The model under review builds one solid part; all positions refer to its coordinate system, in mm. Face numbers are marked on the shaded views. A direction names the side the tool comes from. Coordinates: 2 decimals unless noted, no trailing zeros. Loops run counter-clockwise (first coordinate to the right, second up) from the corner with the lowest first, then second, coordinate; pieces in that order, holes last. Notation, with made-up numbers: M 81,20.25 L 117,20.25 A33 cw 117,58.25 Z; hole C 44.5,76.25 d8. An arc over 180 degrees is marked long. Use one line per item in the form item = value.
```python
from build123d import *

# Parameters (mm, degrees)
SKETCH5_R          = 4.5
CUT_EXTRUDE1_DEPTH = 86
SKETCH6_R          = 13
CUT_EXTRUDE2_DEPTH = 8
CUT_EXTRUDE4_DEPTH = 3
SKETCH9_R          = 1
CUT_EXTRUDE5_DEPTH = 5


with BuildPart() as part:
    # Sketch3 → Revolve1 (revolve)
    with BuildSketch(Plane(origin=(0, 0, 0), x_dir=(0, 0, -1), z_dir=(1, 0, 0))):
        Polygon((-24.411764706, 0), (-24.411764706, -109.5), (-19.411764706, -109.5), (-19.411764706, -94.5), (55.588235294, -94.5), (55.588235294, -109.5), (60.588235294, -109.5), (60.588235294, -84.5), (-14.411764706, -84.5), (-14.411764706, 0), align=None)
    revolve(axis=Axis((0, 0, 33.897058824), (0, 0, -1)))

    # Sketch5 → Cut-Extrude1 (cut, through all)
    with BuildSketch(Plane.XY.offset(24.411764706)):
        Circle(SKETCH5_R)
    extrude(amount=-CUT_EXTRUDE1_DEPTH, mode=Mode.SUBTRACT)

    # Sketch6 → Cut-Extrude2 (cut)
    with BuildSketch(Plane(origin=(0, 0, 14.411764706), x_dir=(-1, 0, 0), z_dir=(0, 0, -1))):
        Circle(SKETCH6_R)
    extrude(amount=-CUT_EXTRUDE2_DEPTH, mode=Mode.SUBTRACT)

    # Sketch8 → Cut-Extrude4 (cut)
    with BuildSketch(Plane(origin=(0, 0, -60.588235294), x_dir=(-1, 0, 0), z_dir=(0, 0, -1))):
        with BuildLine():
            ThreePointArc((11.969710732, 83.647928994), (0, 96.5), (-11.969710732, 83.647928994))
            ThreePointArc((-11.969710732, 83.647928994), (0, 84.5), (11.969710732, 83.647928994))
        make_face()
        with BuildLine():
            ThreePointArc((78.426086849, 31.457890927), (83.571451465, 48.25), (66.456376117, 52.190038067))
            ThreePointArc((66.456376117, 52.190038067), (73.17914662, 42.25), (78.426086849, 31.457890927))
        make_face()
        with BuildLine():
            ThreePointArc((66.456376117, -52.190038067), (83.571451465, -48.25), (78.426086849, -31.457890927))
            ThreePointArc((78.426086849, -31.457890927), (73.17914662, -42.25), (66.456376117, -52.190038067))
        make_face()
        with BuildLine():
            ThreePointArc((-11.969710732, -83.647928994), (0, -96.5), (11.969710732, -83.647928994))
            ThreePointArc((11.969710732, -83.647928994), (0, -84.5), (-11.969710732, -83.647928994))
        make_face()
        with BuildLine():
            ThreePointArc((-78.426086849, -31.457890927), (-83.571451465, -48.25), (-66.456376117, -52.190038067))
            ThreePointArc((-66.456376117, -52.190038067), (-73.17914662, -42.25), (-78.426086849, -31.457890927))
        make_face()
        with BuildLine():
            ThreePointArc((-66.456376117, 52.190038067), (-83.571451465, 48.25), (-78.426086849, 31.457890927))
            ThreePointArc((-78.426086849, 31.457890927), (-73.17914662, 42.25), (-66.456376117, 52.190038067))
        make_face()
    extrude(amount=-CUT_EXTRUDE4_DEPTH, mode=Mode.SUBTRACT)

    # Sketch9 → Cut-Extrude5 (cut)
    with BuildSketch(Plane(origin=(0, 0, -57.588235294), x_dir=(-1, 0, 0), z_dir=(0, 0, -1))):
        with Locations((0, 90.5)):
            Circle(SKETCH9_R)
        with Locations((78.375299042, 45.25)):
            Circle(SKETCH9_R)
        with Locations((78.375299042, -45.25)):
            Circle(SKETCH9_R)
        with Locations((0, -90.5)):
            Circle(SKETCH9_R)
        with Locations((-78.375299042, -45.25)):
            Circle(SKETCH9_R)
        with Locations((-78.375299042, 45.25)):
            Circle(SKETCH9_R)
    extrude(amount=-CUT_EXTRUDE5_DEPTH, mode=Mode.SUBTRACT)


solid = part.part
```
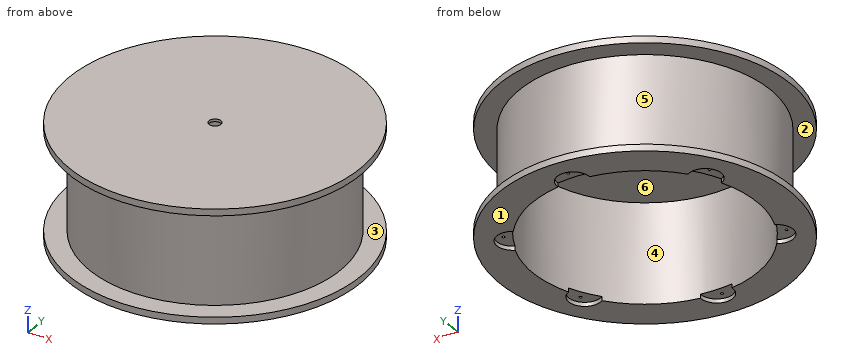
1. Add section C-C (z = -18.5). State the section outline as (x, y) points, then the cut area to 3 significant figures.
Response values:
outline = C 0,0 d189; hole C 0,0 d169
area = 5,620 mm^2
2. Add section D-D (y = 63). State the section outline as (x, z) points.
Response values:
outline = M -89.56,-60.59 L -56.31,-60.59 L -56.31,14.41 L 56.31,14.41 L 56.31,-60.59 L 89.56,-60.59 L 89.56,-55.59 L 70.44,-55.59 L 70.44,19.41 L 89.56,19.41 L 89.56,24.41 L -89.56,24.41 L -89.56,19.41 L -70.44,19.41 L -70.44,-55.59 L -89.56,-55.59 Z
3. Add section B-B (x = -8). State the section outline as (y, z) points.
Response values:
outline = M -109.21,-60.59 L -93.44,-60.59 L -93.44,-57.59 L -84.12,-57.59 L -84.12,14.41 L -10.25,14.41 L -10.25,22.41 L 10.25,22.41 L 10.25,14.41 L 84.12,14.41 L 84.12,-57.59 L 93.44,-57.59 L 93.44,-60.59 L 109.21,-60.59 L 109.21,-55.59 L 94.16,-55.59 L 94.16,19.41 L 109.21,19.41 L 109.21,24.41 L -109.21,24.41 L -109.21,19.41 L -94.16,19.41 L -94.16,-55.59 L -109.21,-55.59 Z
4. Wall thickness on line 1 along Z through (x, y) = (59.5, 88); line 2 along X through (y, z) = (-45, -54); line 3 along Y through (x, z) = (-38, -52): over which ranges is each line inside the solid? List them lowest first. Write a range as from..to.
Response values:
line_1 = -60.59..-55.59, 19.41..24.41
line_2 = -83.1..-79.34, -77.41..-71.52, 71.52..77.41, 79.34..83.1
line_3 = -86.52..-75.47, 75.47..86.52
5. Machinability: for the marked faces 1 and 2, which of the approach directions +Z, -Z, +X, -X, +Y, -Y give a long, thin tool a straight path to every point of the face, cutting with its end or side? Answer none if there is none.
Response values:
face_1 = -Z, +X, -X, +Y, -Y
face_2 = none
6. Add section A-A (y = 0). State the section outline as (x, z) points, then the cut area to 3 significant figures.
Response values:
outline = M -109.5,-60.59 L -84.5,-60.59 L -84.5,14.41 L -13,14.41 L -13,22.41 L -4.5,22.41 L -4.5,24.41 L -109.5,24.41 L -109.5,19.41 L -94.5,19.41 L -94.5,-55.59 L -109.5,-55.59 Z; M 4.5,22.41 L 13,22.41 L 13,14.41 L 84.5,14.41 L 84.5,-60.59 L 109.5,-60.59 L 109.5,-55.59 L 94.5,-55.59 L 94.5,19.41 L 109.5,19.41 L 109.5,24.41 L 4.5,24.41 Z
area = 3,460 mm^2
7. The part is to be moulded in two halves that separate along X. For the marked faces 3, 4, 5 and 6, say which applies: pulls with the +X half, pulls with the -X half, needs draft (parallel to the pull), parting line crosses it, or undercut.
Response values:
face_3 = needs draft
face_4 = undercut
face_5 = parting line crosses it
face_6 = undercut
8. Insertion check: P1, Ø0.6, axis at x = 0, y = 90, coming from the -Z side; P2, Ø2, axis at x = 27, z = -23.5, coming from the +Y side; P3, Ø6, axis at y = -78.5, z = 11.5, coming from the +X side; P4, Ø10.5, axis at x = 4, y = -91, coming from the -Z side. Each pin has a flat end and moves straight along its axis. Give the tip position at first contact, or say it passes through.
Response values:
P1 = -52.59
P2 = 90.85
P3 = 56.83
P4 = -60.59
